Source: CAD feature listing. Evaluate the final solid. Frame: model axes, mm. Face numbers are marked on the shaded views. A direction names the side the tool comes from. Give positions to 0.01 mm unless a question says otherwise; leave off trailing zeros. Write each loop counter-clockwise with the first axis right and the second up, starting at its lowest first coordinate (ties: lowest second). Pieces come first, ordered by that corner, then holes. Notation, with made-up numbers: (1.25, -32.5) -> (30.25, -32.5) arc R27 cw to (30.25, 6.5) -> close; hole circle Ø9 at (63, 48.25). An arc over 180 degrees is marked (long way). Write item = value, one per line.
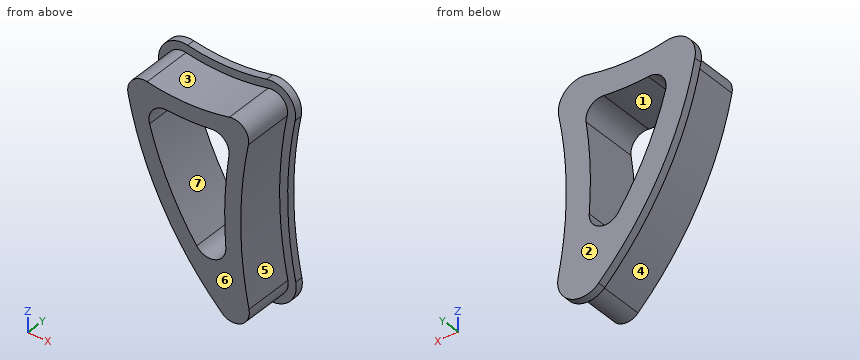
from build123d import *

# Parameters (mm, degrees)
EXTRUDE_1_DEPTH = 6.4
EXTRUDE_2_DEPTH = 1


with BuildPart() as part:
    # 草图1 → 凸台-拉伸1 (new body)
    with BuildSketch(Plane(origin=(0, 0, 0), x_dir=(1, 0, 0), z_dir=(0, 1, 0))):
        with BuildLine():
            ThreePointArc((2.829565104, -15.529906263), (1.88418981, -5.646325328), (2.910376158, 4.229192286))
            ThreePointArc((2.910376158, 4.229192286), (1.906294085, 6.389735523), (-0.452755984, 6.056552897))
            ThreePointArc((-0.452755984, 6.056552897), (-7.914394861, -3.882962322), (-12.140415639, -15.571023149))
            ThreePointArc((-12.140415639, -15.571023149), (-11.58539557, -17.387944), (-9.761966891, -17.92119489))
            ThreePointArc((-9.761966891, -17.92119489), (-4.64989516, -17.37013276), (0.466793237, -17.876538427))
            ThreePointArc((0.466793237, -17.876538427), (2.276755445, -17.336121852), (2.829565104, -15.529906263))
        make_face()
        with BuildLine():
            ThreePointArc((-3.602001562, -0.725023821), (-7.054850169, -6.602735021), (-9.459511378, -12.981391378))
            ThreePointArc((-9.459511378, -12.981391378), (-9.06507879, -14.812553198), (-7.328283633, -15.514175078))
            ThreePointArc((-7.328283633, -15.514175078), (-4.550929201, -15.369896432), (-1.773466789, -15.512081246))
            ThreePointArc((-1.773466789, -15.512081246), (-0.126352502, -14.908348224), (0.411230412, -13.238472884))
            ThreePointArc((0.411230412, -13.238472884), (-0.085305514, -7.64386169), (0.024455921, -2.028331904))
            ThreePointArc((0.024455921, -2.028331904), (-1.293712746, 0.000827838), (-3.602001562, -0.725023821))
        make_face(mode=Mode.SUBTRACT)
    extrude(amount=EXTRUDE_1_DEPTH)

    # 草图2 → 凸台-拉伸2 (add)
    with BuildSketch(Plane(origin=(0, 6.4, 0), x_dir=(1, 0, 0), z_dir=(0, 1, 0))):
        with BuildLine():
            ThreePointArc((3.889844067, 4.027592153), (2.884181446, -5.650415109), (3.810649235, -15.336324425))
            ThreePointArc((3.810649235, -15.336324425), (2.981434747, -18.045647807), (0.266491434, -18.85627267))
            ThreePointArc((0.266491434, -18.85627267), (-4.645529427, -18.370123231), (-9.553118288, -18.899142875))
            ThreePointArc((-9.553118288, -18.899142875), (-12.288261307, -18.09926654), (-13.120791411, -15.373885263))
            ThreePointArc((-13.120791411, -15.373885263), (-8.794151091, -3.407537273), (-1.154854145, 6.768633069))
            ThreePointArc((-1.154854145, 6.768633069), (2.383720959, 7.268407009), (3.889844067, 4.027592153))
        make_face()
        with BuildLine():
            ThreePointArc((0.024455921, -2.028331904), (-0.085305514, -7.64386169), (0.411230412, -13.238472884))
            ThreePointArc((0.411230412, -13.238472884), (-0.126352502, -14.908348224), (-1.773466789, -15.512081246))
            ThreePointArc((-1.773466789, -15.512081246), (-4.550929201, -15.369896432), (-7.328283633, -15.514175078))
            ThreePointArc((-7.328283633, -15.514175078), (-9.06507879, -14.812553198), (-9.459511378, -12.981391378))
            ThreePointArc((-9.459511378, -12.981391378), (-7.054850169, -6.602735021), (-3.602001562, -0.725023821))
            ThreePointArc((-3.602001562, -0.725023821), (-1.293712746, 0.000827838), (0.024455921, -2.028331904))
        make_face(mode=Mode.SUBTRACT)
    extrude(amount=EXTRUDE_2_DEPTH)


solid = part.part
1) Contact query for flat-ended pins moving along their axis: pin 1 (2 mm diameter, centred on y = 4, z = 10.5, fed in from +X); pin 2 (1 mm diameter, centred on y = 5, z = -4, fed in from -X); pin 3 (2 mm diameter, centred on x = -8, y = 1, fed in from +Z). Output: stop coordinate, or through.
Computed:
pin_1 = 2.2
pin_2 = -2.84
pin_3 = 17.77
2) Cut plane A-A (z = 4). Return the cut outline in (x, y), then the cut area to 3 significant figures.
Computed:
outline = (-9.11, 6.4) -> (-7.98, 6.4) -> (-7.98, 0) -> (-5.69, 0) -> (-5.69, 7.4) -> (-9.11, 7.4) -> close; (-0.08, 0) -> (1.92, 0) -> (1.92, 6.4) -> (2.92, 6.4) -> (2.92, 7.4) -> (-0.08, 7.4) -> close
area = 33.9 mm²
3) Draft query along Z for the marked faces 1, 2, 3 and 4. Return one class per face: pulls with the +Z half, pulls with the -Z half, needs draft (parallel to the pull), parting line crosses it, or undercut.
Computed:
face_1 = undercut
face_2 = needs draft
face_3 = pulls with the +Z half
face_4 = pulls with the -Z half
4) Access query for the marked faces 5, 6 and 7. Directions: +Z, -Z, +X, -X, +Y, -Y. A direction counts if a zero-diameter tool reaches every point of the face in a straight line with its end or side. Return the directions, or none.
Computed:
face_5 = +X, -Y
face_6 = +Z, -Z, +X, -X, -Y
face_7 = +Y, -Y
5) Material intervals for L1, parallel to Z at x = -4, y = 4.25; L2, parallel to X at y = 0.5, z = 14; L3, parallel to X at y = 3.75, z = 14.25, sorted ascending.
Computed:
L1 = -2.08 to 1.3, 15.38 to 17.38
L2 = -11.79 to -9.48, 0.37 to 2.55
L3 = -11.85 to -9.4, 0.29 to 2.59
6) Cut plane B-B (x = -4.5). Return the cut outline in (y, z), then the cut area to 3 significant figures.
Computed:
outline = (0, -1.44) -> (6.4, -1.44) -> (6.4, -3.06) -> (7.4, -3.06) -> (7.4, 2.05) -> (0, 2.05) -> close; (0, 15.37) -> (7.4, 15.37) -> (7.4, 18.37) -> (6.4, 18.37) -> (6.4, 17.37) -> (0, 17.37) -> close
area = 43.2 mm²
7) Cut plane C-C (y = 6.75). Return the cut outline in (x, z).
Computed:
outline = (-13.12, 15.37) arc R43 ccw to (-1.15, -6.77) arc R3 ccw to (3.89, -4.03) arc R49 cw to (3.81, 15.34) arc R3 ccw to (0.27, 18.86) arc R24 cw to (-9.55, 18.9) arc R3 ccw to start; hole (-9.46, 12.98) arc R40 ccw to (-3.6, 0.73) arc R2 ccw to (0.02, 2.03) arc R52 cw to (0.41, 13.24) arc R2 ccw to (-1.77, 15.51) arc R27 cw to (-7.33, 15.51) arc R2 ccw to start
8) Cut plane D-D (z = -1.5). Return the cut outline in (x, y), then the cut area to 3 significant figures.
Computed:
outline = (-5.7, 6.4) -> (-4.45, 6.4) -> (-4.45, 0) -> (2.43, 0) -> (2.43, 6.4) -> (3.44, 6.4) -> (3.44, 7.4) -> (-5.7, 7.4) -> close
area = 53.2 mm²
